Study the drawing (mm; zero at the part's minimum x, y, z) and answer. Give positions to 0.01 mm unless a question says otherwise; leave off trailing zeros. Order: outer loops, then holes, each group sorted by start corner. A loop starts at its lowest first (then second) coordinate and runs counter-clockwise, first axis right, second up. Notation, with made-up numbers: (78, 60.5) - (83, 60.5) arc R6 ccw to (83, 70.5) - close; hole circle Ø7 at (-34.75, -32). An arc over 180 degrees is marked (long way). Use CSV: the item, a comma, the result in double quotes.
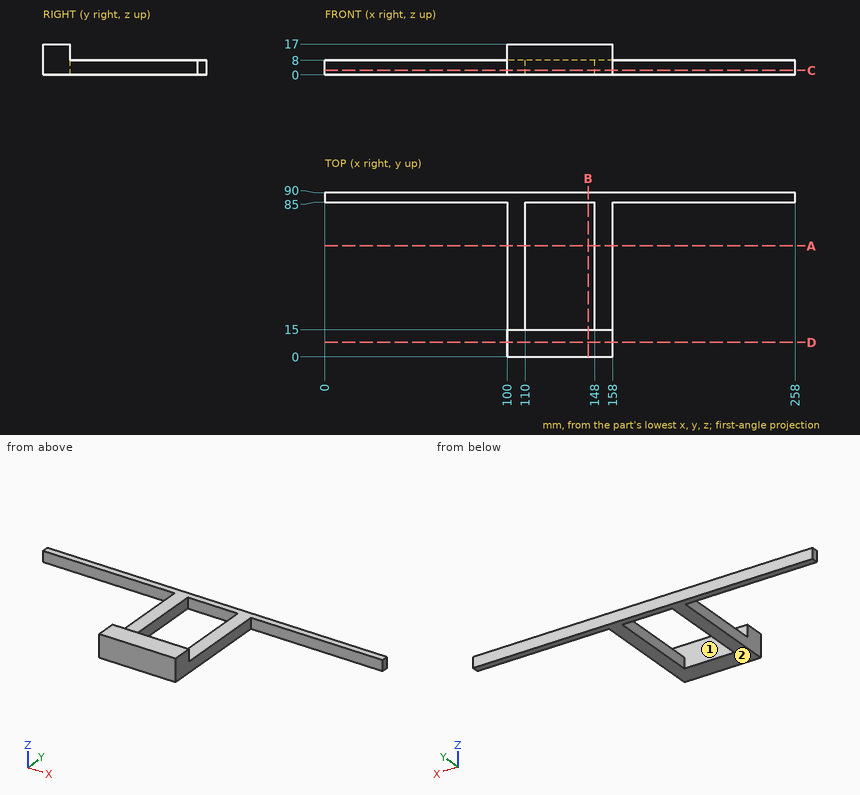
Item 1: The mould has two halves that part along X. Classify the marked faces 1 and 2: +X half, -X half, draft (parallel to the pull), parting line (faces both ways), or undercut.
Taken from the geometry:
face 1,"undercut"
face 2,"draft"
Item 2: Find the intervals of material crossed by line 1 along X through (y, z) = (24.5, 1); line 2 along X through (y, z) = (13, 12); line 3 along Z through (x, y) = (108, 61), in increasing order.
Taken from the geometry:
line 1,"100 to 110, 148 to 158"
line 2,"100 to 158"
line 3,"0 to 8"
Item 3: The part is cut by section A-A (y = 61). Give the vertices of the cut face in (x, z).
Taken from the geometry:
outline,"(100, 0) - (110, 0) - (110, 8) - (100, 8) - close; (148, 0) - (158, 0) - (158, 8) - (148, 8) - close"
Item 4: Each of these flat-tipped pins is pushed along its axis until it touches: pin 1 (8 mm diameter, centred on x = 213, z = 9, fed in from +Y); pin 2 (9 mm diameter, centred on x = 45, z = 2, fed in from -Y); pin 3 (6 mm diameter, centred on y = 51, z = 3.5, fed in from -X); pin 4 (4 mm diameter, centred on y = 48.5, z = 5, fed in from +X). Where does it stop, or does it pass through?
Taken from the geometry:
pin 1,"y = 90"
pin 2,"y = 85"
pin 3,"x = 100"
pin 4,"x = 158"
Item 5: The part is cut by section C-C (z = 2.5). Give the vertices of the cut face in (x, y), and give its area (3 significant figures).
Taken from the geometry:
outline,"(0, 85) - (100, 85) - (100, 0) - (158, 0) - (158, 85) - (258, 85) - (258, 90) - (0, 90) - close; hole (110, 15) - (148, 15) - (148, 85) - (110, 85) - close"
area,"3,560 mm^2"
Item 6: The part is cut by section B-B (x = 144.5). Give the vertices of the cut face in (y, z).
Taken from the geometry:
outline,"(0, 0) - (15, 0) - (15, 17) - (0, 17) - close; (85, 0) - (90, 0) - (90, 8) - (85, 8) - close"
Item 7: The part is cut by section D-D (y = 8). Give the vertices of the cut face in (x, z), and give its area (3 significant figures).
Taken from the geometry:
outline,"(100, 0) - (158, 0) - (158, 17) - (100, 17) - close"
area,"986 mm^2"
